from build123d import *

# Parameters (mm, degrees)
F0_R     = 38.1
F2_R     = 50.8
F4_T     = -2.54
F5_W     = 44.45
F5_H     = 55.88
F6_DEPTH = 25.4
F8_R     = 41.91
F9_DEPTH = 2.54


with BuildPart() as f3:
    # F0 (on Top) → F3 section 0
    with BuildSketch(Plane.XY):
        Circle(F0_R)
    # F2 (on offset) → F3 section 1
    with BuildSketch(Plane.XY.offset(254)):
        Circle(F2_R)
    loft()

    # F4
    f4_openings = [f3.faces().sort_by_distance(p)[0] for p in [
        (0, 0, 254),
    ]]
    offset(amount=F4_T, openings=f4_openings, kind=Kind.INTERSECTION)

    # F5 (on face) → F6 (cut)
    with BuildSketch(Plane(origin=(0, 0, 0), x_dir=(1, 0, 0), z_dir=(0, 0, -1))):
        Rectangle(F5_W, F5_H)
    extrude(amount=-F6_DEPTH, mode=Mode.SUBTRACT)

    # F8 (on offset) → F9 (join)
    with BuildSketch(Plane.XY.offset(127)):
        Circle(F8_R)
    extrude(amount=-F9_DEPTH)


solid = f3.part
Part model, mm, in its own coordinate system. A direction names the side the tool comes from. Give positions to 0.01 mm unless a question says otherwise; leave off trailing zeros. Order: outer loops, then holes, each group sorted by start corner. A loop starts at its lowest first (then second) coordinate and runs counter-clockwise, first axis right, second up. Notation, with made-up numbers: (-4, 34.25) -> (54, 34.25) arc R23 cw to (54, 71.25) -> close; hole circle Ø1 at (-37, 31). An arc over 180 degrees is marked (long way). Use one line per item in the form item = value.
(1) Tool access for faces 5 (the face through (-1, 1, 127)), 6 (the face through (45, -19, 254)), 7 (the face through (0, -31, 2.54)): list every direction of +Z, -Z, +X, -X, +Y, -Y with a clear straight run to the whole face (end or side of a thin tool).
Solution:
face_5 = +Z
face_6 = +Z, +X, -X, +Y, -Y
face_7 = none
(2) Saw through at A-A (x = 0). Write the cut outline in (y, z).
Solution:
outline = (-50.8, 254) -> (-38.1, 0) -> (-27.94, 0) -> (-27.94, 2.54) -> (-35.68, 2.54) -> (-41.78, 124.46) -> (41.78, 124.46) -> (35.68, 2.54) -> (27.94, 2.54) -> (27.94, 0) -> (38.1, 0) -> (50.8, 254) -> (48.26, 254) -> (41.91, 127) -> (-41.91, 127) -> (-48.26, 254) -> close
(3) Drill centre lines: line 1 (Z direction, x = 31, y = 16.5); line 2 (Z direction, x = -8.5, y = 5.5); line 3 (Y direction, x = -29.5, z = 120.5). Where is each one in solid material? Low to high. Write a range as from..to.
Solution:
line_1 = 0..2.54, 124.46..127
line_2 = 124.46..127
line_3 = -32.81..-29.31, 29.31..32.81
(4) Pull direction Z, two halves, no side cores. Call faces 1 (the face through (27, 0, 2.54)), 2 (the face through (25, 1, 0)), 3 (the face through (-28, 0, 2.54)), 4 (the face through (24.26, 38.05, 191.39)): +Z half, -Z half, draft (parallel to the pull), parting line (faces both ways), or undercut.
Solution:
face_1 = undercut
face_2 = -Z half
face_3 = undercut
face_4 = +Z half
(5) Saw through at C-C (z = 174). Write the cut outline in (x, y), then the cut area to 3 significant figures.
Solution:
outline = circle Ø93.6 at (0, 0); hole circle Ø88.51 at (0, 0)
area = 728 mm²
(6) Saw through at B-B (z = 97). Write the cut outline in (x, y), then the cut area to 3 significant figures.
Solution:
outline = circle Ø85.9 at (0, 0); hole circle Ø80.81 at (0, 0)
area = 666 mm²
(7) Flat gauge pins, fed straight in: P1, Ø1, axis at x = 14.5, y = -5.5, coming from the -Z side; P2, Ø2.5, axis at x = -3, y = 33.5, coming from the +Z side; P3, Ø4, axis at y = -7.5, z = 144.5, coming from the +X side. Where does each tip first touch, or does it go through?
Solution:
P1 = 124.46
P2 = 127
P3 = 45.01
